Model file for the job. Use its own axes, mm. Face numbers are marked on the shaded views. A direction names the side the tool comes from. Give positions to 0.01 mm unless a question says otherwise; leave off trailing zeros. Loops run counter-clockwise (first coordinate to the right, second up) from the corner with the lowest first, then second, coordinate; pieces in that order, holes last. Notation, with made-up numbers: M 41,-8.75 L 57,-8.75 A22 cw 57,-0.75 Z; hole C 24.25,-33.75 d11. An arc over 180 degrees is marked long. Use CSV: the item, a comma, the result in double quotes. Start each with the question number.
(1) Slice it at D-D on x = 9. List the corners of the cut face in (y, z), and give its area (3 significant figures).
(2) Two-plate mould, pull along Y, no slides. Class the marked faces 4, 5, 6 and 7: pulls with the +Y half, pulls with the -Y half, needs draft (parallel to the pull), parting line crosses it, or undercut.
(3) Flat gauge pins, fed straight in: P1, Ø5, axis at x = 15, z = 2.5, coming from the +Y side; P2, Ø3, axis at y = 80, z = 3.5, coming from the -X side; P3, Ø3, axis at y = 25.5, z = 6.5, coming from the -X side. Where does each tip first touch, or does it go through?
(4) Wall check: line 1 along Y through (x, z) = (16, 8); line 2 along Y through (x, z) = (20.5, 9.5); line 3 along Y through (x, z) = (21, 7). Give the ranges that are in metal, low to high. Write a range as from..to.
(5) Slice it at C-C on y = 37.5. List the corners of the cut face in (x, z).
(6) Tool access for the marked faces 1, 2 and 3: list every direction of +Z, -Z, +X, -X, +Y, -Y with a clear straight run to the whole face (end or side of a thin tool).
(7) Slice it at A-A on x = 21.5. List the corners of the cut face in (y, z), and give its area (3 significant figures).
Autodesk Fusion 360 part; units mm, degrees
sketch "Sketch1" plane through (0, 0, 0) normal (0, 0, 1) x (1, 0, 0)
  line L0 (0, 0) -> (60, 0)
  line L1 (60, 0) -> (60, 5)
  line L2 (60, 5) -> (0, 5)
  line L3 (0, 5) -> (0, 0)
  line L4 (30, 5) -> (30, 45) construction
  line L5 (30, 5) -> (32.128, 5) construction
  line L6 (32.128, 5) -> (63.7225, 91.8051)
  line L7 (32.128, 5) -> (188.367, 5) construction
  line L8 (30, 5) -> (61.8434, 92.489) construction
  line L9 (30, 5) -> (186.3489, 5) construction
  line L10 (41.3222, 36.1075) -> (16.8902, 45)
  line L11 (30, 45) -> (0, 45) construction
  line L12 (16.8902, 45) -> (15.1801, 40.3015)
  line L13 (32.128, 5) -> (22.128, 5) construction
  line L14 (15.1801, 40.3015) -> (39.6121, 31.409) construction
  line L15 (22.128, 5) -> (32.6609, 33.939)
  line L16 (22.128, 5) -> (52.84, 5) construction
  line L17 (41.3222, 36.1075) -> (61.8434, 92.489)
  line L18 (30, 5) -> (32.128, 5) construction
  line L19 (61.8434, 92.489) -> (63.7225, 91.8051)
  line L20 (15.1801, 40.3015) -> (32.6609, 33.939)
  dimension "d1" = 60
  dimension "d2" = 5
  dimension "d3" = 40
  dimension "d4" = 2.128
  dimension "d5" = 70
  dimension "d6" = 70
  dimension "d7" = 26
  dimension "d8" = 5
  dimension "d9" = 10
  dimension "d10" = 70
  dimension "d11" = 60
extrude "Extrude1" add sketch "Sketch1" along normal blind 10
fillet "Fillet1" radius 5 1 edges at (22.128, 5, 5)
fillet "Fillet2" radius 5 1 edges at (32.128, 5, 5)
fillet "Fillet3" radius 5 1 edges at (32.6609, 33.939, 5)
fillet "Fillet4" radius 5 1 edges at (0, 5, 5)
fillet "Fillet5" radius 5 1 edges at (60, 5, 5)
fillet "Fillet6" radius 5 1 edges at (15.1801, 40.3015, 5)
sketch "Sketch2" plane through (24.8837, -9.0569, 0) normal (-0.9397, 0.342, 0) x (-0.342, -0.9397, 0)
  line L0 (-108.063, 0) -> (-48.063, 0)
  line L1 (-48.063, 0) -> (-48.063, 10)
  line L2 (-48.063, 10) -> (-108.063, 10)
  line L3 (-108.063, 10) -> (-108.063, 0)
  line L4 (-108.063, 5) -> (-101.063, 5) construction
  line L5 (-101.063, 5) -> (-55.063, 5) construction
  circle A0 centre (-55.063, 5) radius 1.75
  circle A1 centre (-101.063, 5) radius 1.75
  dimension "d26" = 7
  dimension "d27" = 46
  dimension "d28" = 3.5
  dimension "d29" = 3.5
extrude "Extrude2" cut sketch "Sketch2" against normal blind 2 contours A0 | A1
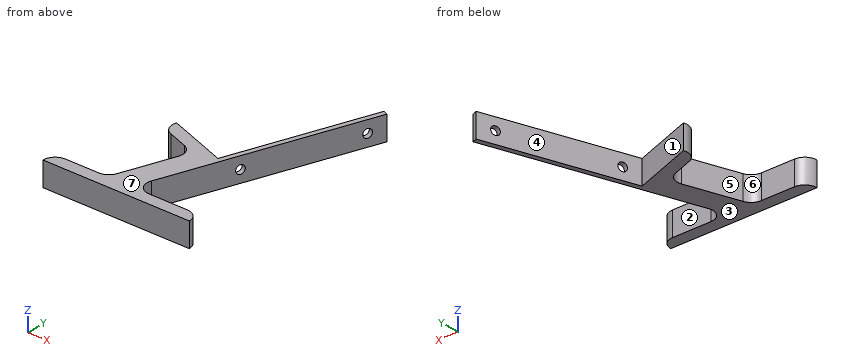
Reply:
1,outline,"M 0,0 L 5,0 L 5,10 L 0,10 Z"
1,area,"50.0 mm^2"
2,face 4,"pulls with the +Y half"
2,face 5,"undercut"
2,face 6,"undercut"
2,face 7,"needs draft"
3,P1,"stops at y = 45"
3,P2,"stops at x = 56.75"
3,P3,"stops at x = 29.04"
4,line 1,"y = 0..5"
4,line 2,"y = 0..5.36, 38.37..43.69"
4,line 3,"y = 0..5.6, 38.18..43.5"
5,outline,"M 22.88,0 L 37.5,0 L 37.5,10 L 22.88,10 Z; M 41.83,0 L 43.96,0 L 43.96,10 L 41.83,10 Z"
6,face 1,"+Z, -Z, +Y"
6,face 2,"+Z, -Z, +X"
6,face 3,"-Z, +X, -X, +Y, -Y"
7,outline,"M 0,0 L 5.91,0 L 5.91,10 L 0,10 Z; M 38,0 L 43.32,0 L 43.32,10 L 38,10 Z"
7,area,"112 mm^2"
